Geometry: final body of the model. Coordinates: model frame, mm. A direction names the side the tool comes from. Give positions to 0.01 mm unless a question says otherwise; leave off trailing zeros. Write each loop counter-clockwise with the first axis right and the second up, starting at its lowest first coordinate (ties: lowest second). Pieces come first, ordered by that corner, then holes. Notation, with made-up numbers: (37, 28.25) -> (90, 28.25) arc R33 ccw to (90, 57.25) -> close; hole circle Ø1 at (10, 26.5). An arc over 180 degrees is marked (long way). Use CSV: the item, a comma, the result in double quotes. Start each with the question number.
1) Material intervals for line 1 (X direction, y = 17.45, z = 0); line 2 (Z direction, x = 60, y = 17); line 3 (Y direction, x = -42, z = 16.5), sorted ascending. Write a range as [from, to].
2) Draft query along Z for faces 4 (the face through (-46.839, -15.145, -21.885)), 5 (the face through (-65.43, 17.52, 2.82)), 6 (the face through (55, 16, 4)). Return one class per face: pulls with the +Z half, pulls with the -Z half, needs draft (parallel to the pull), parting line crosses it, or undercut.
3) Set-up query: faces 1 (the face through (52.465, 18.553, -0.14)), 2 (the face through (-53, 16, 0)), 3 (the face through (-55, 17, 10)). Return all of +Z, -Z, +X, -X, +Y, -Y with unobstructed straight access to the full face (end or side cutting, diameter ignored); none if empty.
4) Section B-B (x = 0). Output: boundary loops of the cut face in (y, z).
5) Section A-A (y = -2.5). Output: boundary loops of the cut face in (x, z).
6) Section C-C (z = 0). Count the separate pieces of the cut face and the enclosed holes in it, plus the area to 3 significant figures.
7) Contact query for flat-ended pins moving along their axis: P1, Ø7.5, axis at x = 5.5, z = -19.5, coming from the +Y side; P2, Ø0.9, axis at x = 53, y = 18, coming from the +Z side; P3, Ø3, axis at y = 13.5, z = -6.5, coming from the -X side; P4, Ø6, axis at y = 18.5, z = -3, coming from the +X side. Output: stop coordinate, or through.
```python
from build123d import *
from OCP.BRepFilletAPI import BRepFilletAPI_MakeChamfer

# Parameters (mm, degrees)
SKETCH1_W                               = 100
SKETCH1_H                               = 50
BOSS_EXTRUDE1_DEPTH                     = 16
SKETCH2_R                               = 20
BOSS_EXTRUDE2_DEPTH                     = 5
BOSS_EXTRUDE3_DEPTH                     = 2
BOSS_EXTRUDE4_DEPTH                     = 3
CHAMFER1_SIZE                           = 5
CHAMFER1_SIZE2                          = 0.881634904
SKETCH3_R                               = 15
BOSS_EXTRUDE5_DEPTH                     = 5
BOSS_EXTRUDE5_TAPER                     = 45
CBORE_FOR_M5_HEX_HEAD_BOLT1_D           = 5.3
CBORE_FOR_M5_HEX_HEAD_BOLT1_DEPTH       = 15
CBORE_FOR_M5_HEX_HEAD_BOLT1_CBORE_D     = 12.24
CBORE_FOR_M5_HEX_HEAD_BOLT1_CBORE_DEPTH = 3.58
CBORE_FOR_M5_HEX_HEAD_BOLT1_TIP         = 1.59228064
CHAMFER2_SIZE                           = 5
FILLET3_R                               = 3


# Read off the part's stored shape, not the designer's step: Boss-Extrude4
with BuildPart() as part:
    # Sketch1 → Boss-Extrude1 (new, symmetric)
    with BuildSketch(Plane(origin=(0, 0, 0), x_dir=(1, 0, 0), z_dir=(0, 1, 0))):
        Rectangle(SKETCH1_W, SKETCH1_H)
    extrude(amount=BOSS_EXTRUDE1_DEPTH, both=True)

    # Sketch2 → Boss-Extrude2 (add)
    with BuildSketch(Plane(origin=(0, 16, 0), x_dir=(1, 0, 0), z_dir=(0, 1, 0))):
        with Locations(Location((0, 0, 0), (0, 0, 90))):
            Circle(SKETCH2_R)
    extrude(amount=BOSS_EXTRUDE2_DEPTH)

    # Sketch2<3> → Boss-Extrude3 (add)
    with BuildSketch(Plane(origin=(0, 16, 0), x_dir=(1, 0, 0), z_dir=(0, 1, 0))):
        with BuildLine():
            Line((-4.084295569, 19.578522153), (-50, 10))
            Line((-50, 10), (-50, -10))
            Line((-50, -10), (-4.084295569, -19.578522153))
            ThreePointArc((-4.084295569, -19.578522153), (-20, 0), (-4.084295569, 19.578522153))
        make_face()
        with BuildLine():
            Line((50, 10), (4.084295569, 19.578522153))
            ThreePointArc((4.084295569, 19.578522153), (15.519115815, 12.615745888), (20, 0))
            ThreePointArc((20, 0), (15.519115815, -12.615745888), (4.084295569, -19.578522153))
            Line((4.084295569, -19.578522153), (50, -10))
            Line((50, -10), (50, 10))
        make_face()
    extrude(amount=BOSS_EXTRUDE3_DEPTH)

    # Boss-Extrude4 outline → Boss-Extrude4 (add)
    with BuildSketch(Plane(origin=(0, 16, 0), x_dir=(1, 0, 0), z_dir=(0, 1, 0))):
        with BuildLine():
            Line((-60, -10), (-50, -10))
            Line((-50, -10), (-50, 10))
            Line((-50, 10), (-60, 10))
            ThreePointArc((-60, 10), (-70, 0), (-60, -10))
        make_face()
        with BuildLine():
            ThreePointArc((60, -10), (70, 0), (60, 10))
            Line((60, 10), (50, 10))
            Line((50, 10), (50, -10))
            Line((50, -10), (60, -10))
        make_face()
    extrude(amount=BOSS_EXTRUDE4_DEPTH)

    # Chamfer1: one chamfer whose edges measure the first distance from different faces: ONE call of the kernel's chamfer builder (chamfer() names one face for all edges)
    chamfer1_edges_1 = [part.edges().sort_by_distance(p)[0] for p in [
        (-50, 19, 0),
    ]]
    chamfer1_side_1 = [part.faces().sort_by_distance(p)[0] for p in [
        (-59.066501411, 19, 0),
    ]]
    chamfer1_edges_2 = [part.edges().sort_by_distance(p)[0] for p in [
        (50, 19, 0),
    ]]
    chamfer1_side_2 = [part.faces().sort_by_distance(p)[0] for p in [
        (59.066501411, 19, 0),
    ]]
    chamfer1 = BRepFilletAPI_MakeChamfer(part.part.solid().wrapped)
    for e in chamfer1_edges_1:
        chamfer1.Add(CHAMFER1_SIZE, CHAMFER1_SIZE2, e.wrapped, chamfer1_side_1[0].wrapped)  # the first distance lies on this face
    for e in chamfer1_edges_2:
        chamfer1.Add(CHAMFER1_SIZE, CHAMFER1_SIZE2, e.wrapped, chamfer1_side_2[0].wrapped)  # the first distance lies on this face
    add(Compound.cast(chamfer1.Shape()), mode=Mode.REPLACE)

    # Sketch3 → Boss-Extrude5 (add)
    with BuildSketch(Plane(origin=(0, 21, 0), x_dir=(1, 0, 0), z_dir=(0, 1, 0))):
        Circle(SKETCH3_R)
    extrude(amount=BOSS_EXTRUDE5_DEPTH, taper=BOSS_EXTRUDE5_TAPER)

    # CBORE for M5 Hex Head Bolt1
    with Locations(Plane(origin=(-60, 19, 0), x_dir=(0, 0, 1), z_dir=(0, 1, 0))):
        with Locations((0, 0), (0, 120)):
            CounterBoreHole(CBORE_FOR_M5_HEX_HEAD_BOLT1_D / 2, CBORE_FOR_M5_HEX_HEAD_BOLT1_CBORE_D / 2, CBORE_FOR_M5_HEX_HEAD_BOLT1_CBORE_DEPTH, depth=CBORE_FOR_M5_HEX_HEAD_BOLT1_DEPTH)
            with Locations((0, 0, -(CBORE_FOR_M5_HEX_HEAD_BOLT1_DEPTH + CBORE_FOR_M5_HEX_HEAD_BOLT1_TIP / 2))):  # 118° drill point
                Cone(0, CBORE_FOR_M5_HEX_HEAD_BOLT1_D / 2, CBORE_FOR_M5_HEX_HEAD_BOLT1_TIP, mode=Mode.SUBTRACT)

    # Chamfer2
    chamfer2_edges = [part.edges().sort_by_distance(p)[0] for p in [
        (50, 0, 25),
        (-50, 0, 25),
        (-50, 0, -25),
        (50, 0, -25),
    ]]
    chamfer(chamfer2_edges, length=CHAMFER2_SIZE)

    # Fillet3
    fillet3_edges = [part.edges().sort_by_distance(p)[0] for p in [
        (-50, -16, 0),
        (-50, 0, 20),
        (-50, 0, -20),
        (50, -16, 0),
        (0, -16, 25),
        (0, -16, -25),
        (47.5, -16, 22.5),
        (-47.5, -16, 22.5),
        (47.5, -16, -22.5),
        (-47.5, -16, -22.5),
        (45, 0, -25),
        (-45, 0, -25),
        (50, 0, 20),
        (50, 0, -20),
        (45, 0, 25),
        (-45, 0, 25),
    ]]
    fillet(fillet3_edges, radius=FILLET3_R)


solid = part.part
```
Answers follow:
1,line 1,"x = [-70, -66.12], [-53.88, 53.88], [66.12, 70]"
1,line 2,"z = [-10, -6.12], [6.12, 10]"
1,line 3,"y = [-16, 16]"
2,face 4,"pulls with the -Z half"
2,face 5,"undercut"
2,face 6,"needs draft"
3,face 1,"+Z, -Z, +Y"
3,face 2,"+Z, -Z, -X, -Y"
3,face 3,"+Z, -X, +Y, -Y"
4,outline,"(-16, -22) arc R3 ccw to (-13, -25) -> (16, -25) -> (16, -20) -> (21, -20) -> (21, -15) -> (26, -10) -> (26, 10) -> (21, 15) -> (21, 20) -> (16, 20) -> (16, 25) -> (-13, 25) arc R3 ccw to (-16, 22) -> close"
5,outline,"(-50, -18.76) arc R3 ccw to (-49.12, -20.88) -> (-45.88, -24.12) arc R3 ccw to (-43.76, -25) -> (43.76, -25) arc R3 ccw to (45.88, -24.12) -> (49.12, -20.88) arc R3 ccw to (50, -18.76) -> (50, 18.76) arc R3 ccw to (49.12, 20.88) -> (45.88, 24.12) arc R3 ccw to (43.76, 25) -> (-43.76, 25) arc R3 ccw to (-45.88, 24.12) -> (-49.12, 20.88) arc R3 ccw to (-50, 18.76) -> close"
6,separate pieces,"3"
6,enclosed holes,"0"
6,area,"3,680 mm^2"
7,P1,"stops at y = 21"
7,P2,"stops at z = 10"
7,P3,"stops at x = -50"
7,P4,"stops at x = 70"
